Geometry: final body of the model. Coordinates: model frame, mm. A direction names the side the tool comes from. Round coordinates to 2 decimals unless told otherwise and drop trailing zeros. Loops run counter-clockwise (first coordinate to the right, second up) from the corner with the lowest first, then second, coordinate; pieces in that order, holes last. Notation, with made-up numbers: (-3.5, -28.5) - (0.5, -28.5) arc R12 cw to (0.5, -17.5) - close; hole circle Ø5 at (16.5, 84.25). An arc over 180 degrees is marked (long way). Answer as a JSON object with one key per item and string values. Group by question number.
Item 1: Draft query along X for faces 1 (the face through (-112.69, -3.75, 157.13)), 2 (the face through (-97, 0, 138)), 3 (the face through (-101, -4, 62)). Return one class per face: released by +X, released by -X, zero draft, split by the parting line, or undercut.
Item 2: First-contact query: pin 1 (10 mm diameter, centred on x = -70, z = 194, fed in from -Y); pin 2 (2 mm diameter, centred on x = -176.5, y = -2, fed in from -Z). Flat tips, straight axial feed; report the tip coordinate or a pass-through.
Item 3: Section D-D (z = 301). Return the cut outline in (x, y).
Item 4: Section C-C (y = 1.5). Return the cut outline in (x, z), plus the area to 3 significant figures.
Item 5: Line query: line 1 (Z direction, x = -100, y = 1.1); line 2 (Y direction, x = -45.5, z = 263.5); line 3 (Z direction, x = -114, y = -3.5). Output: solid intervals per line, ascending.
Item 6: Reachability of faces 4 (the face through (-65.44, -1.97, 114.33)), 5 (the face through (-142.954, 1.972, 117.81)) from +Z, -Z, +X, -X, +Y, -Y: full face, straight path, thin tool, end or side. Return the list, or none.
Autodesk Inventor part; units mm, degrees
ref_plane "YZ Plane" through (0, 0, 0) normal (1, 0, 0) x (0, 1, 0)
ref_plane "XZ Plane" through (0, 0, 0) normal (0, 1, 0) x (-1, 0, 0)
ref_plane "XY Plane" through (0, 0, 0) normal (0, 0, 1) x (1, 0, 0)
sketch "Эскиз1" plane through (0, 0, 0) normal (0, 1, 0) x (-1, 0, 0)
  line L0 (0, 0) -> (200, 0)
  line L1 (200, 0) -> (200, 400)
  line L2 (200, 400) -> (0, 400)
  line L3 (0, 400) -> (0, 0)
  circle A0 centre (100, 100) radius 46.5
  point P0 (100, 0)
  dimension "d0" = 200
  dimension "d1" = 400
  dimension "d2" = 100
  dimension "d3" = 93
extrude "Выдавливание1" add sketch "Эскиз1" along normal blind 4
sketch "Эскиз2" plane through (0, 0, 0) normal (0, -1, 0) x (1, 0, 0)
  circle A0 centre (-100, 100) radius 46.5
  circle A1 centre (-100, 100) radius 58.2755
  circle A2 centre (-100, 100) radius 37.4147
  point P0 (0, 0)
extrude "Выдавливание2" add sketch "Эскиз2" along normal blind 4 contours A0 | A1
chamfer "Фаска1" distance 4 angle 45 1 edges at (-158.2755, 0, 100)
properties part number "типа танк"
Values:
{
 "1": {"face 1": "split by the parting line", "face 2": "undercut", "face 3": "zero draft"},
 "2": {"pin 1": "stops at y = 0", "pin 2": "passes through"},
 "3": {"outline": "(-200, 0) - (0, 0) - (0, 4) - (-200, 4) - close"},
 "4": {"outline": "(-200, 0) - (0, 0) - (0, 400) - (-200, 400) - close; hole circle Ø93 at (-100, 100)", "area": "73,200 mm^2"},
 "5": {"line 1": "z = 0 to 53.5, 146.5 to 400", "line 2": "y = 0 to 4", "line 3": "z = 42.92 to 65.3, 134.7 to 157.08"},
 "6": {"face 4": "+Y, -Y", "face 5": "+Y"}
}
